CAD build for the part. Positions are in the model's coordinates, mm. Coordinates: 2 decimals unless noted, no trailing zeros. Loops run counter-clockwise (first coordinate to the right, second up) from the corner with the lowest first, then second, coordinate; pieces in that order, holes last.
1) Wall check: line 1 along Z through (x, y) = (4.5, 4.1); line 2 along Z through (x, y) = (15, 2) (3 decimals); line 3 along X through (y, z) = (3.1, -4.5). Give the ranges that are in metal, low to high.
2) Saw through at B-B, the plane y = 2.25. Give the number of separate pieces and of enclosed holes in the cut face, and give its area (3 significant figures).
3) Two-plate mould, pull along Z, no slides. Class faces 1 (the cylindrical face through (50.647, 2.788, 48.717)), 2 (the cylindrical face through (3.49, 2.71, -5.61)), 3 (the cylindrical face through (1.353, 2.788, -80.226)): +Z half, -Z half, draft (parallel to the pull), parting line (faces both ways), or undercut.
4) Saw through at A-A, the plane z = -4.5. Write the cut outline in (x, y).
Autodesk Inventor part; units mm, degrees
ref_plane "YZ Plane" through (0, 0, 0) normal (1, 0, 0) x (0, 1, 0)
ref_plane "XZ Plane" through (0, 0, 0) normal (0, 1, 0) x (-1, 0, 0)
ref_plane "XY Plane" through (0, 0, 0) normal (0, 0, 1) x (1, 0, 0)
sketch "スケッチ1" plane through (0, 0, 0) normal (0, 1, 0) x (-1, 0, 0)
  line L0 (0, 0) -> (-52, 0)
  line L1 (-52, 0) -> (-52, -81.5097)
  line L2 (-52, -81.5097) -> (0, -81.5097)
  line L3 (0, -81.5097) -> (0, 0)
  dimension "d0" = 81.5097
  dimension "d1" = 52
extrude "押し出し1" add sketch "スケッチ1" along normal blind 5.5
sketch "スケッチ2" plane through (0, 5.5, 0) normal (0, 1, 0) x (1, 0, 0)
  line L0 (0, 0) -> (52, 0)
  line L1 (52, 81.5097) -> (0, 81.5097)
  line L2 (52, 0) -> (52, 81.5097)
  line L3 (0, 81.5097) -> (0, 0)
  point P0 (4.5, 4.5)
  point P1 (4.5, 77.0097)
  point P2 (47.5, 77.0097)
  point P3 (47.5, 4.5)
  dimension "d4" = 4.5
  dimension "d5" = 4.5
  dimension "d6" = 4.5
  dimension "d7" = 4.5
  dimension "d8" = 4.5
  dimension "d9" = 4.5
  dimension "d10" = 4.5
  dimension "d11" = 4.5
hole "穴1" at (4.5, 5.5, -4.5) at (4.5, 5.5, -77.0097) at (47.5, 5.5, -77.0097) at (47.5, 5.5, -4.5) direction (0, -1, 0) diameter 3 end through all
sketch "スケッチ3" plane through (0, 5.5, 0) normal (0, 1, 0) x (1, 0, 0)
  circle A0 centre (22, 40.7548) radius 15.5
  line L0 (0, 0) -> (52, 0)
  line L1 (52, 81.5097) -> (0, 81.5097)
  line L2 (52, 0) -> (52, 81.5097)
  line L3 (22, 40.7548) -> (35.4234, 33.0048)
  line L4 (22, 40.7548) -> (37.5, 40.7548) construction
  line L5 (22, 40.7548) -> (8.5766, 33.0048)
  line L6 (22, 40.7548) -> (22, 56.2548)
  line L7 (22, 40.7548) -> (37.5, 40.7548) construction
  point P0 (4.5, 0)
  point P1 (47.5, 0)
  point P2 (47.5, 81.5097)
  point P3 (4.5, 81.5097)
  point P4 (52, 4.5)
  point P5 (52, 77.0097)
  dimension "d20" = 31
  dimension "d21" = 81.5097
  dimension "d22" = 40.7548
  dimension "d23" = 30
  dimension "d25" = 90
  dimension "d43" = 120
  dimension "d44" = 120
hole "穴2" at (35.4234, 5.5, -33.0048) at (22, 5.5, -56.2548) at (8.5766, 5.5, -33.0048) direction (0, -1, 0) diameter 3 end through all
sketch "スケッチ4" plane through (0, 5.5, 0) normal (0, 1, 0) x (1, 0, 0)
  line L0 (0, 0) -> (52, 0)
  line L1 (52, 81.5097) -> (0, 81.5097)
  line L2 (52, 0) -> (52, 81.5097)
  point P0 (15, 40.7548)
  point P1 (4.5, 0)
  point P2 (47.5, 0)
  point P3 (47.5, 81.5097)
  point P4 (4.5, 81.5097)
  point P5 (52, 4.5)
  point P6 (52, 77.0097)
  dimension "d33" = 81.5097
  dimension "d34" = 40.7548
  dimension "d35" = 37
hole "穴3" at (15, 5.5, -40.7548) direction (0, -1, 0) diameter 12 end through all
sketch "スケッチ5" plane through (0, 0, 0) normal (0, 0, 1) x (1, 0, 0)
  line L0 (0, 0) -> (0, 5.5)
  line L1 (52, 0) -> (52, 5.5)
  line L2 (0, 0) -> (52, 0)
  line L3 (52, 0) -> (52, 5.5)
  line L4 (52, 5.5) -> (0, 5.5)
  line L5 (0, 5.5) -> (0, 0)
extrude "押し出し2" add sketch "スケッチ5" along normal blind 50
sketch "スケッチ6" plane through (0, 5.5, 0) normal (0, 1, 0) x (1, 0, 0)
  line L0 (0, 81.5097) -> (0, -50)
  circle A0 centre (15, 40.7548) radius 6
  line L1 (52, -50) -> (0, -50)
  point P0 (0, 0)
  point P1 (15, -45.5)
  point P2 (15, -13.07)
  dimension "d47" = 15
  dimension "d48" = 15
  dimension "d49" = 15
  dimension "d57" = 32.43
  dimension "d58" = 4.5
hole "穴4" at (15, 5.5, 45.5) at (15, 5.5, 13.07) direction (0, -1, 0) diameter 3 end through all
sketch "スケッチ7" plane through (0, 5.5, 0) normal (0, 1, 0) x (1, 0, 0)
  circle A0 centre (15, -13.07) radius 1.5
  circle A1 centre (15, -45.5) radius 1.5
  line L0 (0, 81.5097) -> (0, -50)
  point P0 (0, 0)
  point P1 (15, -29.285)
  dimension "d59" = 32.43
  dimension "d60" = 15
  dimension "d61" = 15
  dimension "d62" = 16.215
hole "穴5" at (15, 5.5, 29.285) direction (0, -1, 0) diameter 8 end through all
fillet "フィレット2" radius 4.5 4 edges at (52, 2.75, 50) (0, 2.75, 50) (52, 2.75, -81.5097) (0, 2.75, -81.5097)
equation "\"d22\" = 0.5 * d21"
equation "\"d44\" = d43"
properties part number "ロボット回転t5.5" material "木材 (カエデ材)"
Data:
1. line 1: z = -81.51 to -78.51, -75.51 to -6, -3 to 50
1. line 2: z = -81.51 to -46.755, -34.755 to 11.57, 14.57 to 25.285, 33.285 to 44, 47 to 50
1. line 3: x = 0 to 3, 6 to 46, 49 to 52
2. separate pieces: 1
2. enclosed holes: 11
2. area: 6,590 mm2
3. face 1: +Z half
3. face 2: undercut
3. face 3: -Z half
4. outline: (0, 0) - (3, 0) - (3, 5.5) - (0, 5.5) - close; (6, 0) - (46, 0) - (46, 5.5) - (6, 5.5) - close; (49, 0) - (52, 0) - (52, 5.5) - (49, 5.5) - close
